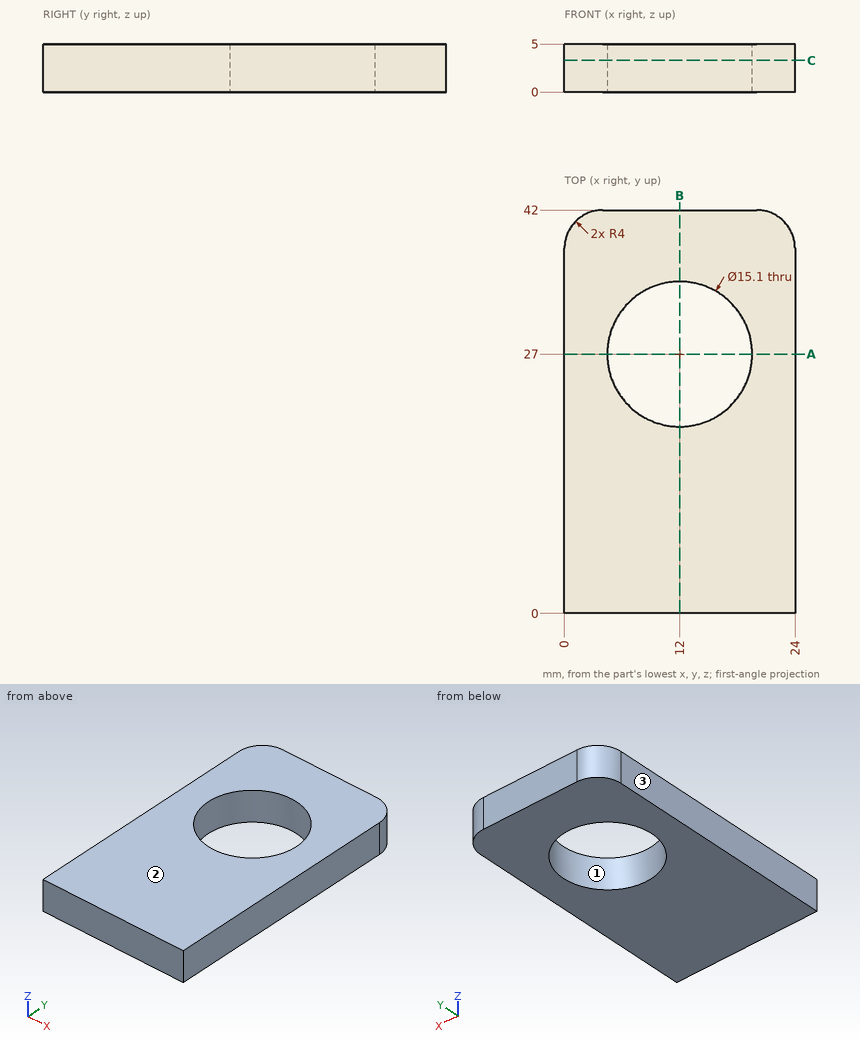
For this review, use the dimensioned drawing (mm, ordinates from the lowest corner) and the shaded views. Round coordinates to 2 decimals unless told otherwise and drop trailing zeros. Order: outer loops, then holes, each group sorted by start corner. A loop starts at its lowest first (then second) coordinate and runs counter-clockwise, first axis right, second up. Notation, with made-up numbers: M 89,18.25 L 112,18.25 A28 cw 112,46.25 Z; hole C -35.75,-29 d3. An arc over 180 degrees is marked long. Use a Markdown table: item, result.
1) Insertion check: pin 1 (2 mm diameter, centred on x = 10.5, y = 19.5, fed in from -Z). The pin has a flat end and moves straight along its axis. Give the tip position at first contact, or say it passes through.
Report:
| item | result |
|---|---|
| pin 1 | z = 0 |
2) Wall thickness on line 1 along Y through (x, z) = (12, 3.25); line 2 along Y through (x, z) = (15.5, 0.35); line 3 along X through (y, z) = (32, 4.45): over which ranges is each line inside the solid? List them lowest first. Write a range as [from, to].
Report:
| item | result |
|---|---|
| line 1 | [0, 19.45], [34.55, 42] |
| line 2 | [0, 20.31], [33.69, 42] |
| line 3 | [0, 6.34], [17.66, 24] |
3) Consider section A-A (y = 27). Write out the cut boundary in (x, z).
Report:
| item | result |
|---|---|
| outline | M 0,0 L 4.45,0 L 4.45,5 L 0,5 Z; M 19.55,0 L 24,0 L 24,5 L 19.55,5 Z |
4) Draft analysis for pull direction X (two halves, no side actions). For the marked faces 1, 2 and 3, state which applies: released by +X, released by -X, zero draft, split by the parting line, or undercut.
Report:
| item | result |
|---|---|
| face 1 | undercut |
| face 2 | zero draft |
| face 3 | released by -X |
5) Consider section B-B (x = 12). Write out the cut boundary in (y, z), then the cut area to 4 significant figures.
Report:
| item | result |
|---|---|
| outline | M 0,0 L 19.45,0 L 19.45,5 L 0,5 Z; M 34.55,0 L 42,0 L 42,5 L 34.55,5 Z |
| area | 134.5 mm^2 |
6) Consider section C-C (z = 3.3). Write out the cut boundary in (x, y), then the cut area to 3 significant figures.
Report:
| item | result |
|---|---|
| outline | M 0,0 L 24,0 L 24,38 A4 ccw 20,42 L 4,42 A4 ccw 0,38 Z; hole C 12,27 d15.1 |
| area | 822 mm^2 |
